from build123d import *

# Parameters (mm, degrees)
SKETCH1_R           = 45
SKETCH1_R_2         = 25
BOSS_EXTRUDE1_DEPTH = 8
CHAMFER1_SIZE       = 3
CUT_EXTRUDE1_START  = -17
CUT_EXTRUDE1_DEPTH  = 18
CIRPATTERN1_COUNT   = 12


with BuildPart() as part:
    # Sketch1 → Boss-Extrude1 (new body, symmetric)
    with BuildSketch(Plane.XY):
        Circle(SKETCH1_R)
        Circle(SKETCH1_R_2, mode=Mode.SUBTRACT)
    extrude(amount=BOSS_EXTRUDE1_DEPTH, both=True)

    # Chamfer1
    chamfer1_edges = [part.edges().sort_by_distance(p)[0] for p in [
        (-25, 0, 8),
    ]]
    chamfer(chamfer1_edges, length=CHAMFER1_SIZE)

    # Sketch2 → Cut-Extrude1 (cut)
    with BuildSketch(Plane.XY.offset(8).offset(CUT_EXTRUDE1_START)):
        with BuildLine():
            Line((0, 45), (0, 34))
            Line((0, 34), (-21.215955949, 39.684798263))
            ThreePointArc((-21.215955949, 39.684798263), (-10.935814514, 43.650978923), (0, 45))
        make_face()
    cut_extrude1 = extrude(amount=CUT_EXTRUDE1_DEPTH, mode=Mode.SUBTRACT)

    # CirPattern1: Cut-Extrude1 ×12 about axis
    cirpattern1_axis = Axis((0, 0, 0), (0, 0, 1))
    for i in range(1, CIRPATTERN1_COUNT):
        add(cut_extrude1.rotate(cirpattern1_axis, i * 360 / CIRPATTERN1_COUNT), mode=Mode.SUBTRACT)


solid = part.part
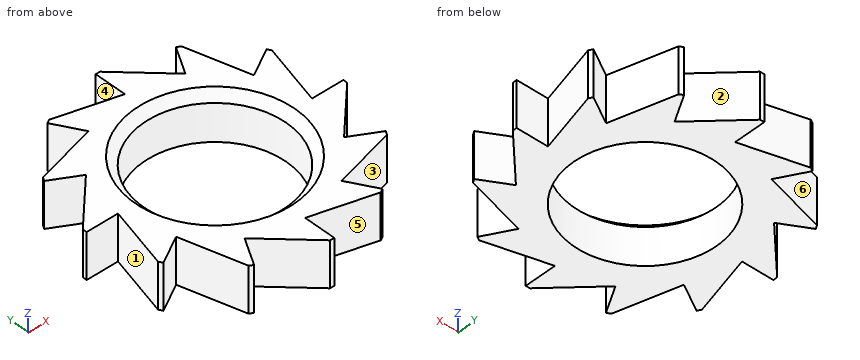
Source: CAD feature listing. Evaluate the final solid. Frame: model axes, mm. Face numbers are marked on the shaded views. A direction names the side the tool comes from. Coordinates: 2 decimals unless noted, no trailing zeros. Order: outer loops, then holes, each group sorted by start corner. A loop starts at its lowest first (then second) coordinate and runs counter-clockwise, first axis right, second up.
Item 1: Cut plane A-A (x = 36). Return loops of the section in (y, z), plus the area to 3 significant figures.
Output values:
outline: (-24.35, -8) - (-20.78, -8) - (-20.78, 8) - (-24.35, 8) - close; (-10.44, -8) - (0, -8) - (0, 8) - (-10.44, 8) - close; (7.46, -8) - (20.78, -8) - (20.78, 8) - (7.46, 8) - close
area: 437 mm2
Item 2: Material intervals for line 1 (Y direction, x = -17.5, z = -4); line 2 (X direction, y = -18, z = 0); line 3 (X direction, y = -3, z = 1.25), sorted ascending.
Output values:
line 1: y = -30.31 to -17.85, 17.85 to 29.31, 30.31 to 38.69
line 2: x = -38.82 to -31.18, -29.18 to -17.35, 17.35 to 31.18
line 3: x = -34.8 to -24.82, 24.82 to 43.44
Item 3: Set-up query: the marked faces 1, 2 and 3. Return all of +Z, -Z, +X, -X, +Y, -Y with unobstructed straight access to the full face (end or side cutting, diameter ignored); none if empty.
Output values:
face 1: +Z, -Z, -X
face 2: +Z, -Z, +Y
face 3: +Z, -Z, +X
Item 4: First-contact query: P1, Ø8, axis at x = 8.5, z = -0.5, coming from the +Y side; P2, Ø4, axis at y = -20.5, z = -5, coming from the -X side; P3, Ø9, axis at x = 41.5, z = 0.5, coming from the +Y side. Flat tips, straight axial feed; report the tip coordinate or a pass-through.
Output values:
P1: stops at y = 41.94
P2: stops at x = -39.68
P3: stops at y = 22.5
Item 5: Pull-direction query (Y, two-part tool) for the marked faces 4, 5 and 6; classes: pulls with the +Y half, pulls with the -Y half, needs draft (parallel to the pull), parting line crosses it, or undercut.
Output values:
face 4: needs draft
face 5: pulls with the -Y half
face 6: undercut
Item 6: Cut plane B-B (x = 19). Count the separate pieces of the cut face and the enclosed holes in it, plus the area to 3 significant figures.
Output values:
separate pieces: 3
enclosed holes: 0
area: 555 mm2
